Can you work these out from the model? Positions are in its coordinate system, mm. Face numbers are marked on the shaded views. Coordinates: 2 decimals unless noted, no trailing zeros. Loops run counter-clockwise (first coordinate to the right, second up) from the corner with the lowest first, then second, coordinate; pieces in that order, holes last.
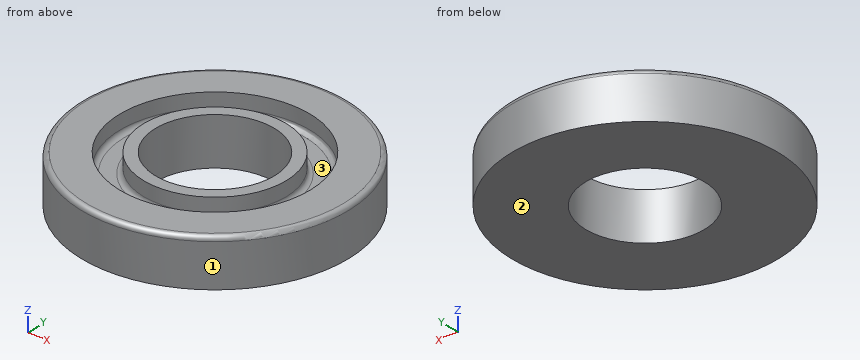
```python
from build123d import *

# Parameters (mm, degrees)
F0_R     = 17.78
F0_R_2   = 7.9375
F1_DEPTH = 6.35
F2_R     = 12.7
F2_R_2   = 9.525
F3_DEPTH = 2.54
F4_R     = 0.635


with BuildPart() as f1:
    # F0 (on Top) → F1 (new body)
    with BuildSketch(Plane.XY):
        Circle(F0_R)
        Circle(F0_R_2, mode=Mode.SUBTRACT)
    extrude(amount=F1_DEPTH)

    # F2 (on face) → F3 (cut)
    with BuildSketch(Plane.XY.offset(6.35)):
        Circle(F2_R)
        Circle(F2_R_2, mode=Mode.SUBTRACT)
    extrude(amount=-F3_DEPTH, mode=Mode.SUBTRACT)

    # F4
    f4_edges = [f1.edges().sort_by_distance(p)[0] for p in [
        (-17.78, 0, 6.35),
        (-12.7, 0, 3.81),
        (-9.525, 0, 3.81),
    ]]
    fillet(f4_edges, radius=F4_R)


solid = f1.part
```
Item 1: We'd pull the mould along Y, two halves only. Please class the marked faces 1, 2 and 3: +Y half, -Y half, draft (parallel to the pull), parting line (faces both ways), or undercut.
Results are:
face 1: parting line
face 2: draft
face 3: undercut
Item 2: Suppose I cut it at C-C, the plane z = 5. Count the separate pieces of the cut face and the enclosed holes in it, plus the area to 3 significant figures.
Results are:
separate pieces: 2
enclosed holes: 2
area: 574 mm2
Item 3: I'm going to push flat-ended pins straight in: P1, Ø12.5, axis at x = 0, y = 0, coming from the -Z side; P2, Ø1.5, axis at y = -3.5, z = 5.5, coming from the -X side. Where does each tip first touch, or does it pass through?
Results are:
P1: passes through
P2: stops at x = -17.57
Item 4: Suppose I cut it at D-D, the plane z = 1.75. Please give me the cut outline in (x, y) (1 decimal), plus the area to 3 significant figures.
Results are:
outline: circle Ø35.6 at (0, 0); hole circle Ø15.9 at (0, 0)
area: 795 mm2
Item 5: I need wall thicknesses on line 1 along Y through (x, z) = (0, 4.5) (1 decimal); line 2 along Y through (x, z) = (0, 4.25); line 3 along X through (y, z) = (-4, 4). Which ranges of each line are inside material? Lowest first, please.
Results are:
line 1: y = -17.8 to -12.7, -9.5 to -7.9, 7.9 to 9.5, 12.7 to 17.8
line 2: y = -17.78 to -12.67, -9.56 to -7.94, 7.94 to 9.56, 12.67 to 17.78
line 3: x = -17.32 to -11.86, -8.84 to -6.86, 6.86 to 8.84, 11.86 to 17.32
